Design review of the part built by this model. Coordinates are the model's own, in mm. A direction names the side the tool comes from. Coordinates: 2 decimals unless noted, no trailing zeros. Answer in a Markdown table with one row per item.
from build123d import *

# Parameters (mm, degrees)
F0_W      = 30
F0_H      = 30
F1_DEPTH  = 15
F2_R      = 2
F3_R      = 2
F10_D     = 2
F10_DEPTH = 0.508
F10_TIP   = 0.600860619
F11_D     = 2
F11_DEPTH = 0.508
F11_TIP   = 0.600860619
F12_D     = 2
F12_DEPTH = 0.508
F12_TIP   = 0.600860619
F13_D     = 2
F13_DEPTH = 0.508
F13_TIP   = 0.600860619
F14_D     = 2
F14_DEPTH = 0.508
F14_TIP   = 0.600860619
F15_D     = 2
F15_DEPTH = 0.508
F15_TIP   = 0.600860619


with BuildPart() as f1:
    # F0 (on Front) → F1 (new body, symmetric)
    with BuildSketch(Plane.XZ):
        with Locations((-1.0603153623, 0.943120569)):
            Rectangle(F0_W, F0_H)
    extrude(amount=F1_DEPTH, both=True)

    # F2
    f2_edges = [f1.edges().sort_by_distance(p)[0] for p in [
        (-1.060315, -15, 15.943121),
    ]]
    fillet(f2_edges, radius=F2_R)

    # F3
    f3_edges = [f1.edges().sort_by_distance(p)[0] for p in [
        (13.939685, 1, 15.943121),
        (-1.060315, 15, 15.943121),
        (-16.060315, 1, 15.943121),
        (-16.060315, 15, 0.943121),
        (13.939685, 15, 0.943121),
        (13.939685, -15, -0.056879),
        (-16.060315, 0, -14.056879),
        (-1.060315, 15, -14.056879),
        (13.939685, 0, -14.056879),
        (-1.060315, -15, -14.056879),
        (-16.060315, -15, -0.056879),
    ]]
    fillet(f3_edges, radius=F3_R)

    # F10
    with Locations(Plane.XZ.offset(15)):
        with Locations((-1.0603153623, 0.943120569)):
            Hole(F10_D / 2, depth=F10_DEPTH)
            with Locations((0, 0, -(F10_DEPTH + F10_TIP / 2))):  # 118° drill point
                Cone(0, F10_D / 2, F10_TIP, mode=Mode.SUBTRACT)

    # F11
    with Locations(Plane.XY.offset(15.943120569)):
        with Locations((-11.0603153623, 10), (-1.0603153623, 0), (8.9396846377, 10), (8.9396846377, -10), (-11.0603153623, -10)):
            Hole(F11_D / 2, depth=F11_DEPTH)
            with Locations((0, 0, -(F11_DEPTH + F11_TIP / 2))):  # 118° drill point
                Cone(0, F11_D / 2, F11_TIP, mode=Mode.SUBTRACT)

    # F12
    with Locations(Plane(origin=(0, 15, 0), x_dir=(-1, 0, 0), z_dir=(0, 1, 0))):
        with Locations((-8.9396846377, 10.943120569), (-8.9396846377, 0.943120569), (-8.9396846377, -9.056879431), (11.0603153623, -9.056879431), (11.0603153623, 0.943120569), (11.0603153623, 10.943120569)):
            Hole(F12_D / 2, depth=F12_DEPTH)
            with Locations((0, 0, -(F12_DEPTH + F12_TIP / 2))):  # 118° drill point
                Cone(0, F12_D / 2, F12_TIP, mode=Mode.SUBTRACT)

    # F13
    with Locations(Plane(origin=(0, 0, -14.056879431), x_dir=(1, 0, 0), z_dir=(0, 0, -1))):
        with Locations((8.9396846377, 10), (-11.0603153623, -10)):
            Hole(F13_D / 2, depth=F13_DEPTH)
            with Locations((0, 0, -(F13_DEPTH + F13_TIP / 2))):  # 118° drill point
                Cone(0, F13_D / 2, F13_TIP, mode=Mode.SUBTRACT)

    # F14
    with Locations(Plane.YZ.offset(13.9396846377)):
        with Locations((-10, 10.943120569), (-10, -9.056879431), (10, -9.056879431), (10, 10.943120569)):
            Hole(F14_D / 2, depth=F14_DEPTH)
            with Locations((0, 0, -(F14_DEPTH + F14_TIP / 2))):  # 118° drill point
                Cone(0, F14_D / 2, F14_TIP, mode=Mode.SUBTRACT)

    # F15
    with Locations(Plane(origin=(-16.0603153623, 0, 0), x_dir=(0, -1, 0), z_dir=(-1, 0, 0))):
        with Locations((-10, 10.943120569), (0, 0.943120569), (10, -9.056879431)):
            Hole(F15_D / 2, depth=F15_DEPTH)
            with Locations((0, 0, -(F15_DEPTH + F15_TIP / 2))):  # 118° drill point
                Cone(0, F15_D / 2, F15_TIP, mode=Mode.SUBTRACT)


solid = f1.part
(1) Draft analysis for pull direction X (two halves, no side actions). For faces 1 (the cylindrical face through (-15.803, 9.263, 11.619)), 2 (the cylindrical face through (-1.522, -14.742, 0.056)), 3 (the conical face through (12.935, -10.128, -8.94)), 4 (the conical face through (8.8, -10.11, 14.94)), state which applies: pulls with the +X half, pulls with the -X half, needs draft (parallel to the pull), parting line crosses it, or undercut.
Return value:
| item | result |
|---|---|
| face 1 | needs draft |
| face 2 | undercut |
| face 3 | pulls with the +X half |
| face 4 | undercut |
(2) For line 1 along Z through (x, y) = (13.65, -10); line 2 along Z through (x, y) = (13.55, -10); line 3 along X through (y, z) = (-3, -12.25), list the stretches that pass through material, from the lowest coordinate up. Write a range as from..to.
Return value:
| item | result |
|---|---|
| line 1 | z = -13.09..-10.06, -8.06..9.94, 11.94..14.98 |
| line 2 | z = -13.24..-10.06, -8.06..9.94, 11.94..15.13 |
| line 3 | x = -16.05..13.93 |
(3) Insertion check: pin 1 Ø1.8 at (x, z) = (-1.06, 0.94) entering from -Y; pin 2 Ø1.8 at (x, y) = (-11.06, 10) entering from +Z. Each pin has a flat end and moves straight along its axis. Give the tip position at first contact, or say it passes through.
Return value:
| item | result |
|---|---|
| pin 1 | stops at y = -14.43 |
| pin 2 | stops at z = 15.38 |
(4) For faces 5 (the cylindrical face through (-11.797, 14.742, -8.381)), 6 (the cylindrical face through (-15.803, -0.217, -0.033)), 7 (the conical face through (12.94, 9.98, 11.12)), 8 (the cylindrical face through (9.07, -9.01, 15.69)), 9 (the cylindrical face through (13.34, -14.43, 1.13)), list the 3-axis set-ups (+Z, -Z, +X, -X, +Y, -Y) from which the entire face can be reached by the end or side of a thin tool; tool diameter is ignored.
Return value:
| item | result |
|---|---|
| face 5 | +Y |
| face 6 | -X |
| face 7 | +X |
| face 8 | +Z |
| face 9 | +Z, -Z, +X, -Y |
